Autodesk Inventor part; units mm, degrees
ref_plane "YZ Plane" through (0, 0, 0) normal (1, 0, 0) x (0, 1, 0)
ref_plane "XZ Plane" through (0, 0, 0) normal (0, 1, 0) x (-1, 0, 0)
ref_plane "XY Plane" through (0, 0, 0) normal (0, 0, 1) x (1, 0, 0)
sketch "Sketch1" plane through (0, 0, 0) normal (0, 0, 1) x (1, 0, 0)
  circle A0 centre (0, 0) radius 41.148
  dimension "d0" = 82.296
extrude "Extrusion1" add sketch "Sketch1" against normal blind 5.969
sketch "Sketch2" plane through (0, 0, 0) normal (0, 0, 1) x (1, 0, 0)
  circle A0 centre (0, 0) radius 17.018
  dimension "d3" = 34.036
extrude "Extrusion2" cut sketch "Sketch2" against normal blind 5.969
sketch "Sketch3" plane through (0, 0, 0) normal (0, 0, 1) x (1, 0, 0)
  circle A0 centre (0, 36.449) radius 2.3813
  circle A1 centre (-31.5658, 18.2245) radius 2.3813
  circle A2 centre (-31.5658, -18.2245) radius 2.3813
  circle A3 centre (0, -36.449) radius 2.3813
  circle A4 centre (31.5658, -18.2245) radius 2.3813
  circle A5 centre (31.5658, 18.2245) radius 2.3813
  point P0 (0, 0)
  dimension "d6" = 4.7625
  dimension "d9" = 360
extrude "Extrusion3" cut sketch "Sketch3" against normal blind 5.969
properties part number "retainRing4_4"
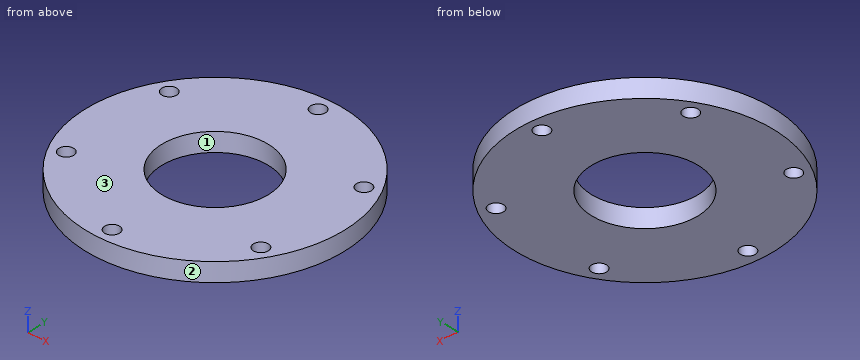
The model under review builds one solid part; all positions refer to its coordinate system, in mm. Face numbers are marked on the shaded views. Round coordinates to 2 decimals unless told otherwise and drop trailing zeros. Order: outer loops, then holes, each group sorted by start corner. A loop starts at its lowest first (then second) coordinate and runs counter-clockwise, first axis right, second up. Notation, with made-up numbers: (57.5, 11.5) -> (98.5, 11.5) arc R11 ccw to (98.5, 24.5) -> close; hole circle Ø6 at (-35.75, 68). An arc over 180 degrees is marked (long way). Return JSON: item names as keys, results as strings.
1. Take a section at D-D (x = -10). Write out the cut boundary in (y, z).
Answer block:
{"outline": "(-39.91, -5.97) -> (-13.77, -5.97) -> (-13.77, 0) -> (-39.91, 0) -> close; (13.77, -5.97) -> (39.91, -5.97) -> (39.91, 0) -> (13.77, 0) -> close"}
2. Take a section at A-A (y = 0). Write out the cut boundary in (x, z).
Answer block:
{"outline": "(-41.15, -5.97) -> (-17.02, -5.97) -> (-17.02, 0) -> (-41.15, 0) -> close; (17.02, -5.97) -> (41.15, -5.97) -> (41.15, 0) -> (17.02, 0) -> close"}
3. Take a section at B-B (x = 0). Write out the cut boundary in (y, z), then the cut area to 3 significant figures.
Answer block:
{"outline": "(-41.15, -5.97) -> (-38.83, -5.97) -> (-38.83, 0) -> (-41.15, 0) -> close; (-34.07, -5.97) -> (-17.02, -5.97) -> (-17.02, 0) -> (-34.07, 0) -> close; (17.02, -5.97) -> (34.07, -5.97) -> (34.07, 0) -> (17.02, 0) -> close; (38.83, -5.97) -> (41.15, -5.97) -> (41.15, 0) -> (38.83, 0) -> close", "area": "231 mm²"}
4. The part is to be moulded in two halves that separate along Y. For the marked faces 1, 2 and 3, say which applies: +Y half, -Y half, draft (parallel to the pull), parting line (faces both ways), or undercut.
Answer block:
{"face 1": "undercut", "face 2": "parting line", "face 3": "draft"}
5. Insertion check: P1, Ø3, axis at x = 0, y = 36.449, coming from the -Z side; P2, Ø1, axis at x = -27, z = -1.5, coming from the +Y side; P3, Ø1, axis at y = 7.5, z = -4.5, coming from the -X side. Each pin has a flat end and moves straight along its axis. Give the tip position at first contact, or say it passes through.
Answer block:
{"P1": "passes through", "P2": "stops at y = 31.48", "P3": "stops at x = -40.55"}
6. For L1, parallel to Y at x = 0, z = -4.4; L2, parallel to X at y = 18, z = -4.3; L3, parallel to X at y = -10.5, z = -3.35, list the stretches that pass through material, from the lowest coordinate up. Write a range as [from, to].
Answer block:
{"L1": "y = [-41.15, -38.83], [-34.07, -17.02], [17.02, 34.07], [38.83, 41.15]", "L2": "x = [-37, -33.94], [-29.2, 29.2], [33.94, 37]", "L3": "x = [-39.79, -13.39], [13.39, 39.79]"}
7. Take a section at C-C (z = -2.2). Write out the cut boundary in (x, y), then the cut area to 3 significant figures.
Answer block:
{"outline": "circle Ø82.3 at (0, 0); hole circle Ø4.76 at (-31.57, -18.22); hole circle Ø4.76 at (-31.57, 18.22); hole circle Ø34.04 at (0, 0); hole circle Ø4.76 at (0, -36.45); hole circle Ø4.76 at (0, 36.45); hole circle Ø4.76 at (31.57, -18.22); hole circle Ø4.76 at (31.57, 18.22)", "area": "4,300 mm²"}
